Check sheet for the modelled part. Datum: model origin and axes. Units: mm. A direction names the side the tool comes from. Give positions to 0.01 mm unless a question says otherwise; leave off trailing zeros. Write each loop counter-clockwise with the first axis right and the second up, starting at its lowest first coordinate (ties: lowest second). Pieces come first, ordered by that corner, then holes. Notation, with made-up numbers: (34.25, 5) -> (43.25, 5) arc R14 cw to (43.25, 18) -> close; hole circle Ø2 at (37, -22.75). An arc over 180 degrees is marked (long way). Return JSON: item names as keys, results as strings.
from build123d import *

# Parameters (mm, degrees)
FILLET1_R          = 2.54
SKETCH2_R          = 7.62
CUT_EXTRUDE1_DEPTH = 6.35
SKETCH3_R          = 1.5875
CUT_EXTRUDE2_DEPTH = 6.35


with BuildPart() as part:
    # Sketch1 → Revolve1 (revolve)
    with BuildSketch(Plane.XY):
        Polygon((0, 0), (0, 11.1125), (15.24, 11.1125), (15.24, 26.9875), (322.199, 26.9875), (322.199, 25.1714), (325.374, 25.1714), (325.374, 28.8925), (334.899, 28.8925), (334.899, 15.875), (348.107, 15.875), (348.107, 0), align=None)
    revolve(axis=Axis((0, 0, 0), (1, 0, 0)))

    # Fillet1
    fillet1_edges = [part.edges().sort_by_distance(p)[0] for p in [
        (15.24, -26.9875, 0),
    ]]
    fillet(fillet1_edges, radius=FILLET1_R)

    # Sketch2 → Cut-Extrude1 (cut)
    with BuildSketch(Plane.ZY):
        Circle(SKETCH2_R)
    extrude(amount=-CUT_EXTRUDE1_DEPTH, mode=Mode.SUBTRACT)

    # Sketch3 → Cut-Extrude2 (cut)
    with BuildSketch(Plane.ZY.offset(-6.35)):
        Circle(SKETCH3_R)
    extrude(amount=-CUT_EXTRUDE2_DEPTH, mode=Mode.SUBTRACT)


solid = part.part
(1) Thickness scan on L1, parallel to X at y = 18.5, z = -15; L2, parallel to X at y = 0, z = 25; L3, parallel to Z at x = 158.5, y = -4. Record the ranges inside material, lowest first.
Reply:
{"L1": "15.24 to 334.9", "L2": "15.3 to 334.9", "L3": "-26.69 to 26.69"}
(2) Release check for a two-part mould opening along Z. For faces 1 (the flat face through (0, -2, 8)), 2 (the cylindrical face through (3.13, -7.44, -1.65)), 3 (the cylindrical face through (323.809, 23.252, -9.641)), 4 (the flat face through (6.35, 0, 2)) record: pulls with the +Z half, pulls with the -Z half, needs draft (parallel to the pull), parting line crosses it, or undercut.
Reply:
{"face 1": "needs draft", "face 2": "undercut", "face 3": "parting line crosses it", "face 4": "undercut"}
(3) Set-up check for faces 5 (the flat face through (334.899, 12, -12)), 6 (the flat face through (322.199, 18, -18)), 7 (the cylindrical face through (172.12, -19.89, 18.24)): record each of +Z, -Z, +X, -X, +Y, -Y from which the full face is reachable in a straight line by a thin tool's end or side.
Reply:
{"face 5": "+X", "face 6": "none", "face 7": "-X"}
(4) Depth check by flat-ended pin: pin 1 Ø9 at (y, z) = (0, 0) entering from -X; pin 2 Ø3 at (x, z) = (214, 5) entering from +Y; pin 3 Ø12 at (x, y) = (238.5, 16.5) entering from -Z; pin 4 Ø17 at (y, z) = (1, 1) entering from -X. Enter the tip coordinate at first touch or a pass-through.
Reply:
{"pin 1": "x = 6.35", "pin 2": "y = 26.76", "pin 3": "z = -24.86", "pin 4": "x = 0"}
(5) Cross-section at A-A on x = 303.5. Enter the section's corners in (y, z) (1 decimal).
Reply:
{"outline": "circle Ø54 at (0, 0)"}
